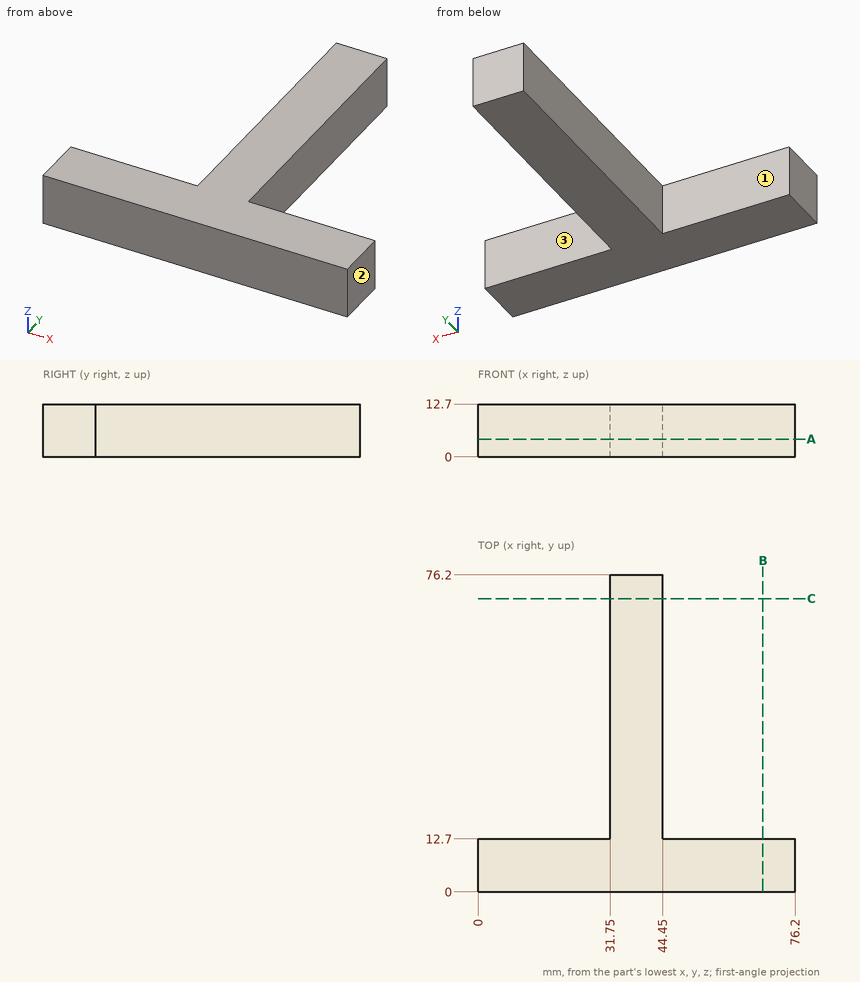
Could you check a few things on this drawing? It's one solid part, dimensions in mm from its lowest x, y, z. A direction names the side the tool comes from. Coordinates: 2 decimals unless noted, no trailing zeros. Write each loop counter-clockwise with the first axis right and the second up, starting at its lowest first coordinate (ties: lowest second). Pieces come first, ordered by that corner, then holes. Notation, with made-up numbers: (55.5, 22) - (113.5, 22) arc R17 ccw to (113.5, 36) - close; hole circle Ø5 at (53.5, 53). An arc over 180 degrees is marked (long way). Return JSON: item names as keys, results as strings. Group by question number.
Item 1: If we section it at B-B (x = 68.5): Write out the boundary of the cut face in (y, z).
Item 2: I'm going to push flat-ended pins straight in: pin 1 Ø1.5 at (y, z) = (24, 3.5) entering from +X; pin 2 Ø2 at (y, z) = (56.5, 11) entering from -X; pin 3 Ø4 at (x, z) = (66, 8.5) entering from +Y. Where does each tip first touch, or does it pass through?
Item 3: Which directions (+Z, -Z, +X, -X, +Y, -Y) give clear straight access to the entire face, cutting with the end or side of a thin tool? Please do the marked faces 1, 2 and 3.
Item 4: Please list where these lines run through material, in increasing order: probe 1 along Y at (x, z) = (48, 12); probe 2 along X at (y, z) = (48.5, 10.5).
Item 5: If we section it at C-C (y = 70.5): Write out the boundary of the cut face in (x, z).
Item 6: If we section it at A-A (z = 4.25): Write out the boundary of the cut face in (x, y).
Return value:
{
 "1": {"outline": "(0, 0) - (12.7, 0) - (12.7, 12.7) - (0, 12.7) - close"},
 "2": {"pin 1": "stops at x = 44.45", "pin 2": "stops at x = 31.75", "pin 3": "stops at y = 12.7"},
 "3": {"face 1": "+Z, -Z, -X, +Y", "face 2": "+Z, -Z, +X, +Y, -Y", "face 3": "+Z, -Z, +X, +Y"},
 "4": {"probe 1": "y = 0 to 12.7", "probe 2": "x = 31.75 to 44.45"},
 "5": {"outline": "(31.75, 0) - (44.45, 0) - (44.45, 12.7) - (31.75, 12.7) - close"},
 "6": {"outline": "(0, 0) - (76.2, 0) - (76.2, 12.7) - (44.45, 12.7) - (44.45, 76.2) - (31.75, 76.2) - (31.75, 12.7) - (0, 12.7) - close"}
}
